Geometry: final body of the model. Coordinates: model frame, mm. A direction names the side the tool comes from. Give positions to 0.01 mm unless a question says otherwise; leave off trailing zeros. Write each loop counter-clockwise with the first axis right and the second up, starting at its lowest first coordinate (ties: lowest second). Pieces come first, ordered by that corner, then holes. Notation, with made-up numbers: (82.25, 14) -> (92.25, 14) arc R9 cw to (92.25, 25) -> close; hole circle Ø9 at (44.5, -5.5). An arc over 180 degrees is marked (long way). Answer as a JSON object with one key per item and string values. Group by question number.
(1) Material intervals for probe 1 along X at (y, z) = (-0.5, 1.4); probe 2 along X at (y, z) = (-1.5, 0.4); probe 3 along Y at (x, z) = (-10, 1.2), sorted ascending.
(2) Set-up query: faces 4 (the face through (-2.74, -12.35, 1.14)), 5 (the face through (0.04, -0.02, 0.76)), 6 (the face through (0, 0, 1.524)). Return all of +Z, -Z, +X, -X, +Y, -Y with unobstructed straight access to the full face (end or side cutting, diameter ignored); none if empty.
(3) Section query C-C on y = 5. Output: boundary loops of the cut face in (x, z).
(4) Section query A-A on y = 0. Output: boundary loops of the cut face in (x, z).
(5) Section query D-D on x = 4.5. Output: boundary loops of the cut face in (y, z), plus the area to 3 significant figures.
(6) Draft query along X for faces 1 (the face through (0, 0, 0.254)), 2 (the face through (-12.5, 3.2, 0.762)), 3 (the face through (-1.82, 13.85, 0.38)). Return one class per face: +X half, -X half, draft (parallel to the pull), parting line (faces both ways), or undercut.
from build123d import *

# Parameters (mm, degrees)
F0_R     = 12.65
F1_DEPTH = 1.524
F2_R     = 13.97
F3_DEPTH = 0.762
F4_W     = 5.08
F4_H     = 1.524
F6_W     = 5.08000508
F6_H     = 1.5265774739
F7_DEPTH = 0.254
F8_R     = 0.25399


# Not quite as in the source:
# - a fillet or chamfer is up to 0.001 mm smaller than in the source, because OpenCascade refuses the exact size


with BuildPart() as f1:
    # F0 (on Top) → F1 (new body)
    with BuildSketch(Plane.XY):
        Circle(F0_R)
    extrude(amount=F1_DEPTH)

    # F2 (on Top) → F3 (join)
    with BuildSketch(Plane.XY):
        Circle(F2_R)
    extrude(amount=F3_DEPTH)

    # F4 (on Front) → F5 (revolve, cut)
    with BuildSketch(Plane.XZ):
        Rectangle(F4_W, F4_H)
    revolve(axis=Axis((0, 0, -0.762), (-1, 0, 0)), mode=Mode.SUBTRACT)

    # F6 (on Top) → F7 (join)
    with BuildSketch(Plane.XY):
        Rectangle(F6_W, F6_H)
    extrude(amount=F7_DEPTH)

    # F8 (radius 0.254 in the source; OpenCascade refuses exactly that, so slightly less here)
    f8_edges = [f1.edges().sort_by_distance(p)[0] for p in [
        (0, 0.763289, 0.254),
        (0, -0.763289, 0.254),
    ]]
    fillet(f8_edges, radius=F8_R)


solid = f1.part
Answer list:
{
 "1": {"probe 1": "-12.64 to 12.64", "probe 2": "-13.89 to 13.89", "probe 3": "-7.75 to 7.75"},
 "2": {"face 4": "+Z", "face 5": "none", "face 6": "+Z, +X, -X, +Y, -Y"},
 "3": {"outline": "(-13.04, 0) -> (13.04, 0) -> (13.04, 0.76) -> (11.62, 0.76) -> (11.62, 1.52) -> (-11.62, 1.52) -> (-11.62, 0.76) -> (-13.04, 0.76) -> close"},
 "4": {"outline": "(-13.97, 0) -> (13.97, 0) -> (13.97, 0.76) -> (12.65, 0.76) -> (12.65, 1.52) -> (-12.65, 1.52) -> (-12.65, 0.76) -> (-13.97, 0.76) -> close; hole (-2.54, 0.25) -> (2.54, 0.25) -> (2.54, 0.76) -> (-2.54, 0.76) -> close"},
 "5": {"outline": "(-13.23, 0) -> (13.23, 0) -> (13.23, 0.76) -> (11.82, 0.76) -> (11.82, 1.52) -> (-11.82, 1.52) -> (-11.82, 0.76) -> (-13.23, 0.76) -> close", "area": "38.2 mm2"},
 "6": {"face 1": "undercut", "face 2": "draft", "face 3": "parting line"}
}
